Check sheet for the modelled part. Datum: model origin and axes. Units: mm. Give positions to 0.01 mm unless a question says otherwise; leave off trailing zeros. Order: outer loops, then holes, each group sorted by start corner. A loop starts at its lowest first (then second) coordinate and runs counter-clockwise, first axis right, second up. Notation, with made-up numbers: (46, -4.5) -> (71, -4.5) arc R14 cw to (71, 19.5) -> close; hole circle Ø8 at (22, -27). An arc over 180 degrees is marked (long way). Write each question's results on one line, items separated by ' | '.
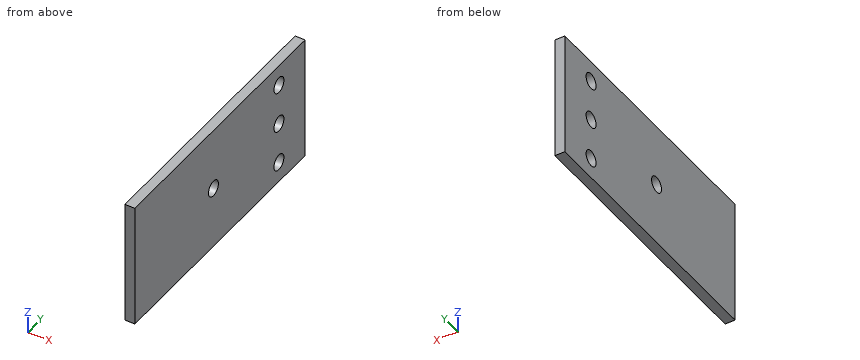
Autodesk Fusion 360 part; units mm, degrees
sketch "Sketch1" plane through (0, 0, 0) normal (1, 0, 0) x (0, 1, 0)
  line L0 (0, 0) -> (82.55, 0)
  line L1 (82.55, 0) -> (82.55, 38.1)
  line L2 (82.55, 38.1) -> (0, 38.1)
  line L3 (0, 38.1) -> (0, 0)
  dimension "d1" = 82.55
  dimension "d2" = 38.1
extrude "Extrude1" add sketch "Sketch1" along normal blind 3.048
sketch "Sketch2" plane through (3.048, 0, 0) normal (1, 0, 0) x (0, 1, 0)
  line L0 (0, 38.1) -> (0, 0)
  line L1 (0, 0) -> (82.55, 0)
  line L2 (82.55, 0) -> (82.55, 38.1)
  line L3 (82.55, 38.1) -> (0, 38.1)
  line L4 (0, 0) -> (38.1, 0)
  line L5 (38.1, 0) -> (38.1, 19.05)
  line L6 (38.1, 19.05) -> (0, 19.05)
  line L7 (0, 19.05) -> (0, 0)
  dimension "d5" = 38.1
  dimension "d6" = 19.05
hole "Hole1" at (3.048, 38.1, 19.05) direction (-1, 0, 0) diameter 4.826 depth 9.652 tip angle 118
sketch "Sketch3" plane through (3.048, 0, 0) normal (1, 0, 0) x (0, 1, 0)
  circle A0 centre (38.1, 19.05) radius 2.413
  line L0 (0, 38.1) -> (0, 0)
  line L1 (0, 0) -> (82.55, 0)
  line L2 (82.55, 0) -> (82.55, 38.1)
  line L3 (82.55, 38.1) -> (0, 38.1)
  line L4 (82.55, 0) -> (69.85, 0)
  line L5 (69.85, 0) -> (69.85, 6.35)
  line L6 (69.85, 6.35) -> (82.55, 6.35)
  line L7 (82.55, 6.35) -> (82.55, 0)
  dimension "d10" = 12.7
  dimension "d11" = 6.35
hole "Hole2" at (3.048, 69.85, 6.35) direction (-1, 0, 0) diameter 4.826 depth 3.048 tip angle 118
sketch "Sketch4" plane through (3.048, 0, 0) normal (1, 0, 0) x (0, 1, 0)
  circle A0 centre (69.85, 6.35) radius 2.413
  circle A1 centre (38.1, 19.05) radius 2.413
  line L0 (0, 38.1) -> (0, 0)
  line L1 (0, 0) -> (82.55, 0)
  line L2 (82.55, 0) -> (82.55, 38.1)
  line L3 (82.55, 38.1) -> (0, 38.1)
  line L4 (82.55, 0) -> (69.85, 0)
  line L5 (69.85, 0) -> (69.85, 19.05)
  line L6 (69.85, 19.05) -> (82.55, 19.05)
  line L7 (82.55, 19.05) -> (82.55, 0)
  dimension "d15" = 12.7
  dimension "d16" = 19.05
hole "Hole3" at (3.048, 69.85, 19.05) direction (-1, 0, 0) diameter 4.826 depth 3.048 tip angle 118
sketch "Sketch5" plane through (3.048, 0, 0) normal (1, 0, 0) x (0, 1, 0)
  circle A0 centre (69.85, 19.05) radius 2.413
  circle A1 centre (69.85, 6.35) radius 2.413
  circle A2 centre (38.1, 19.05) radius 2.413
  line L0 (0, 38.1) -> (0, 0)
  line L1 (0, 0) -> (82.55, 0)
  line L2 (82.55, 0) -> (82.55, 38.1)
  line L3 (82.55, 38.1) -> (0, 38.1)
  line L4 (82.55, 0) -> (69.85, 0)
  line L5 (69.85, 0) -> (69.85, 31.75)
  line L6 (69.85, 31.75) -> (82.55, 31.75)
  line L7 (82.55, 31.75) -> (82.55, 0)
  dimension "d20" = 12.7
  dimension "d21" = 31.75
hole "Hole4" at (3.048, 69.85, 31.75) direction (-1, 0, 0) diameter 4.826 depth 3.048 tip angle 118
1. Section check B-B on z = 31.75. Record the cut outline in (x, y), then the cut area to 3 significant figures.
Verdict:
outline: (0, 0) -> (3.05, 0) -> (3.05, 67.44) -> (0, 67.44) -> close; (0, 72.26) -> (3.05, 72.26) -> (3.05, 82.55) -> (0, 82.55) -> close | area: 237 mm^2
2. Section check C-C on x = 1.85. Record the cut outline in (y, z), then the cut area to 3 significant figures.
Verdict:
outline: (0, 0) -> (82.55, 0) -> (82.55, 38.1) -> (0, 38.1) -> close; hole circle Ø4.83 at (38.1, 19.05); hole circle Ø4.83 at (69.85, 6.35); hole circle Ø4.83 at (69.85, 19.05); hole circle Ø4.83 at (69.85, 31.75) | area: 3,070 mm^2
3. Section check D-D on y = 69.85. Record the cut outline in (x, z).
Verdict:
outline: (0, 0) -> (3.05, 0) -> (3.05, 3.94) -> (0, 3.94) -> close; (0, 8.76) -> (3.05, 8.76) -> (3.05, 16.64) -> (0, 16.64) -> close; (0, 21.46) -> (3.05, 21.46) -> (3.05, 29.34) -> (0, 29.34) -> close; (0, 34.16) -> (3.05, 34.16) -> (3.05, 38.1) -> (0, 38.1) -> close
4. Gauge pin test, flat end, axial feed: pin 1 Ø4 at (y, z) = (69.85, 19.05) entering from +X. Record the tip position at first contact, or that the pin passes through.
Verdict:
pin 1: passes through
5. Material ranges on probe 1 along Z at (x, y) = (0.9, 69.85); probe 2 along Y at (x, z) = (1.25, 31.75); probe 3 along Y at (x, z) = (1.65, 19.05), recorded low to high. Write a range as from..to.
Verdict:
probe 1: z = 0..3.94, 8.76..16.64, 21.46..29.34, 34.16..38.1 | probe 2: y = 0..67.44, 72.26..82.55 | probe 3: y = 0..35.69, 40.51..67.44, 72.26..82.55
6. Section check A-A on y = 38.1. Record the cut outline in (x, z).
Verdict:
outline: (0, 0) -> (3.05, 0) -> (3.05, 16.64) -> (0, 16.64) -> close; (0, 21.46) -> (3.05, 21.46) -> (3.05, 38.1) -> (0, 38.1) -> close
